For this review, take the finished solid that the model builds, in its own axes (mm). A direction names the side the tool comes from. Round coordinates to 2 decimals unless told otherwise and drop trailing zeros. Loops run counter-clockwise (first coordinate to the right, second up) from the corner with the lowest first, then second, coordinate; pieces in that order, holes last. Notation, with made-up numbers: (-29, 70.5) -> (-17, 70.5) arc R14 ccw to (-17, 90.5) -> close; hole circle Ø5 at (-12, -5). An arc over 180 degrees is marked (long way). Write each question's results on one line, items separated by ' | '.
```python
from build123d import *

# Parameters (mm, degrees)
ESBO_O2_R                = 4.5
RESSALTO_EXTRUS_O1_DEPTH = 16.2
ESBO_O3_R                = 2.1
CORTE_EXTRUS_O2_DEPTH    = 13.2
ESBO_O5_R                = 0.75
RESSALTO_EXTRUS_O2_DEPTH = 0.7
ESBO_O11_R               = 0.8
CORTE_EXTRUS_O3_DEPTH    = 0.7
ESBO_O8_R                = 0.275
RESSALTO_EXTRUS_O3_DEPTH = 13


with BuildPart() as part:
    # Esboço2 → Ressalto-extrusão1 (new body)
    with BuildSketch(Plane(origin=(0, 0, 0), x_dir=(1, 0, 0), z_dir=(0, 1, 0))):
        with Locations(Location((0, 0, 0), (0, 0, 270))):
            Circle(ESBO_O2_R)
    extrude(amount=RESSALTO_EXTRUS_O1_DEPTH)

    # Esboço3 → Corte-extrusão2 (cut)
    with BuildSketch(Plane(origin=(0, 16.2, 0), x_dir=(1, 0, 0), z_dir=(0, 1, 0))):
        with Locations(Location((0, 0, 0), (0, 0, 270))):
            Circle(ESBO_O3_R)
    extrude(amount=-CORTE_EXTRUS_O2_DEPTH, mode=Mode.SUBTRACT)

    # Esboço5 → Corte-Revolução1 (revolve, cut)
    with BuildSketch(Plane(origin=(0, 0, 0), x_dir=(0, 0, -1), z_dir=(1, 0, 0)), mode=Mode.PRIVATE) as corte_revolu_o1_sk:
        with Locations((4.7, 14.62)):
            Circle(ESBO_O5_R)
    revolve(corte_revolu_o1_sk.sketch.rotate(Axis((0, 16.2, 0), (0, -1, 0)), 180), axis=Axis((0, 16.2, 0), (0, -1, 0)), mode=Mode.SUBTRACT)

    # Esboço12 → Ressalto-extrusão2 (add)
    with BuildSketch(Plane.XZ):
        with BuildLine():
            Line((3.342126206, -3.174726822), (3.73922223, -3.491162716))
            Line((3.73922223, -3.491162716), (4.237785194, -2.865515075))
            Line((4.237785194, -2.865515075), (3.84068917, -2.549079181))
            ThreePointArc((3.84068917, -2.549079181), (-3.605005954, 2.87273912), (3.342126206, -3.174726822))
        make_face()
    extrude(amount=RESSALTO_EXTRUS_O2_DEPTH)

    # Esboço11 → Corte-extrusão3 (cut)
    with BuildSketch(Plane(origin=(0, 0, 0), x_dir=(1, 0, 0), z_dir=(0, 1, 0))):
        with Locations(Location((2.54, 0, 0), (0, 0, 270))):
            Circle(ESBO_O11_R)
        with Locations(Location((0, -2.54, 0), (0, 0, 270))):
            Circle(ESBO_O11_R)
        with Locations(Location((-2.54, 0, 0), (0, 0, 270))):
            Circle(ESBO_O11_R)
        with Locations(Location((0, 2.54, 0), (0, 0, 270))):
            Circle(ESBO_O11_R)
    extrude(amount=-CORTE_EXTRUS_O3_DEPTH, mode=Mode.SUBTRACT)

    # Esboço8 → Ressalto-extrusão3 (add)
    with BuildSketch(Plane(origin=(0, 0, 0), x_dir=(-1, 0, 0), z_dir=(0, -1, 0))):
        with Locations(Location((-2.54, 0, 0), (0, 0, 270))):
            Circle(ESBO_O8_R)
        with Locations(Location((0, 2.54, 0), (0, 0, 270))):
            Circle(ESBO_O8_R)
        with Locations(Location((2.54, 0, 0), (0, 0, 270))):
            Circle(ESBO_O8_R)
        with Locations(Location((0, -2.54, 0), (0, 0, 270))):
            Circle(ESBO_O8_R)
    extrude(amount=RESSALTO_EXTRUS_O3_DEPTH)

    # Esboço15 → Corte-Revolução2 (revolve, cut)
    with BuildSketch(Plane(origin=(0, 0, 0), x_dir=(0, 0, -1), z_dir=(1, 0, 0))):
        Polygon((4.5, 16.20375847), (4.5, 15.70375847), (4.000000985, 16.204750978), align=None)
    revolve(axis=Axis((0, 16.204750978, 0), (0, 1, 0)), mode=Mode.SUBTRACT)


solid = part.part
```
1. Draft analysis for pull direction X (two halves, no side actions). For faces 4 (the face through (1.352, 15.521, 4.292)), 5 (the face through (-2, 16.2, 2)), 6 (the face through (0.04, -0.35, 1.74)), 7 (the face through (-3.32, -0.35, -0.17)), state which applies: released by +X, released by -X, zero draft, split by the parting line, or undercut.
Values found:
face 4: split by the parting line | face 5: zero draft | face 6: undercut | face 7: undercut
2. Tool access review of faces 1 (the face through (0.631, 9.692, 2.003)), 2 (the face through (-3.5, -0.3, 3)), 3 (the face through (-0.49, -0.35, -3.17)): name each direction out of +Z, -Z, +X, -X, +Y, -Y from which nothing blocks a thin tool from reaching the whole face with its end or side.
Values found:
face 1: +Y | face 2: +Y, -Y | face 3: -Y
3. Consider section A-A (y = -10). State the section outline as (x, z) points (3 decimals).
Values found:
outline: circle Ø0.55 at (-2.54, 0); circle Ø0.55 at (0, -2.54); circle Ø0.55 at (0, 2.54); circle Ø0.55 at (2.54, 0)
4. To check wall thickness, follow probe 1 along X at (y, z) = (-0.15, 0) (3 decimals); probe 2 along X at (y, z) = (7, 0); probe 3 along Y at (x, z) = (-3.25, 1.25). State the ranges of each line that lie inside material, in increasing order.
Values found:
probe 1: x = -4.61 to -3.34, -2.815 to -2.265, -1.74 to 1.74, 2.265 to 2.815, 3.34 to 4.61 | probe 2: x = -4.5 to -2.1, 2.1 to 4.5 | probe 3: y = -0.7 to 16.2
5. For pin 1 (1.3 mm diameter, centred on x = -0.5, z = 2, fed in from -Y); pin 2 (1.5 mm diameter, centred on x = -3.5, y = 4.5, fed in from +Z); pin 3 (4 mm diameter, centred on y = 13, z = -1.5, fed in from -X); pin 4 (3 mm diameter, centred on x = 3, y = -4, fed in from -Z) (3 decimals), all flat-tipped, find the tip position at first contact; note any pin that passes through.
Values found:
pin 1: stops at y = -13 | pin 2: stops at z = 3.56 | pin 3: stops at x = -4.5 | pin 4: stops at z = -0.275
